Read the model definition and answer for the solid it produces. Units are mm, in the model's axes. A direction names the side the tool comes from. Give positions to 0.01 mm unless a question says otherwise; leave off trailing zeros. Loops run counter-clockwise (first coordinate to the right, second up) from the corner with the lowest first, then second, coordinate; pieces in that order, holes last. Notation, with made-up numbers: (-4, -31.5) - (48, -31.5) arc R8 cw to (48, -17.5) - close; hole circle Ø8 at (57, 73). An arc over 180 degrees is marked (long way). Put each result on its own line as item: value. Start each with the question number.
1. For faces 1 (the flat face through (3, 1.6, -2.1)), 2 (the flat face through (1, 4, -3)), 3 (the flat face through (53, 3, -17.46)), determine the directions among +Z, -Z, +X, -X, +Y, -Y from which every point of the face is accessible in a straight line to the end or side of a thin tool.
2. Consider L1, parallel to Y at x = 52.8, z = -15.81; L2, parallel to X at y = 5.5, z = -15; L3, parallel to X at y = 0.75, z = -13. Determine where each line is inside the solid, lowest interval first. Write a range as from..to.
3. A cutting plane is placed at C-C, the plane y = 0.5. Determine the outline of the cut face in (x, z).
4. A cutting plane is placed at B-B, the plane y = 3. Determine the outline of the cut face in (x, z).
5. Given pin 1 Ø3.5 at (y, z) = (3, -1.5) entering from +X; pin 2 Ø6 at (x, z) = (33, -4) entering from +Y; pin 3 Ø2 at (y, z) = (4.5, -8) entering from -X; pin 4 Ø1.2 at (y, z) = (3.5, -16) entering from -X, each flat-ended and moving along its own axis, determine where each tip first touches the part or whether it passes through.
6. A cutting plane is placed at D-D, the plane x = 34. Determine the outline of the cut face in (y, z).
7. For a pull along Y with two mould halves and no side action, classify faces 4 (the flat face through (51, 2, -15)), 5 (the flat face through (25, 0, -8)), 6 (the cylindrical face through (1.48, 2.98, -0.65)) as released by +Y, released by -Y, zero draft, split by the parting line, or undercut.
8. A cutting plane is placed at A-A, the plane z = -15.81. Determine the outline of the cut face in (x, y).
```python
from build123d import *

# Parameters (mm, degrees)
BOSS_EXTRUDE1_DEPTH = 6
SKETCH3_R           = 1
CUT_EXTRUDE1_DEPTH  = 59


with BuildPart() as part:
    # Sketch1 → Boss-Extrude1 (new body)
    with BuildSketch(Plane(origin=(0, 0, 0), x_dir=(1, 0, 0), z_dir=(0, 1, 0))):
        with BuildLine():
            Line((0, 6.17), (0, 0))
            Line((0, 0), (3, 0))
            Line((3, 0), (3, 4.33))
            ThreePointArc((3, 4.33), (3.292893219, 5.037106781), (4, 5.33))
            Line((4, 5.33), (52, 9.54))
            ThreePointArc((52, 9.54), (53.414213562, 10.125786438), (54, 11.54))
            Line((54, 11.54), (54, 17.46))
            Line((54, 17.46), (51, 17.46))
            Line((51, 17.46), (51, 13.38))
            ThreePointArc((51, 13.38), (50.707106781, 12.672893219), (50, 12.38))
            Line((50, 12.38), (2, 8.17))
            ThreePointArc((2, 8.17), (0.585786438, 7.584213562), (0, 6.17))
        make_face()
    extrude(amount=BOSS_EXTRUDE1_DEPTH)

    # Sketch3 → Cut-Extrude1 (cut)
    with BuildSketch(Plane(origin=(0, 0, 0), x_dir=(0, 0, -1), z_dir=(1, 0, 0))):
        with Locations(Location((15.81, 3, 0), (0, 0, 180))):
            Circle(SKETCH3_R)
        with BuildLine():
            Line((1.65, 4), (3.65, 4))
            ThreePointArc((3.65, 4), (4.65, 3), (3.65, 2))
            Line((3.65, 2), (1.65, 2))
            ThreePointArc((1.65, 2), (0.65, 3), (1.65, 4))
        make_face()
    extrude(amount=CUT_EXTRUDE1_DEPTH, mode=Mode.SUBTRACT)


solid = part.part
```
Return value:
1. face 1: +Z, +X, +Y, -Y
1. face 2: +X, -X
1. face 3: -Z, +X, -X, +Y, -Y
2. L1: y = 0..2, 4..6
2. L2: x = 51..54
2. L3: x = 50.92..54
3. outline: (0, -6.17) arc R2 ccw to (2, -8.17) - (50, -12.38) arc R1 cw to (51, -13.38) - (51, -17.46) - (54, -17.46) - (54, -11.54) arc R2 ccw to (52, -9.54) - (4, -5.33) arc R1 cw to (3, -4.33) - (3, 0) - (0, 0) - close
4. outline: (0, -6.17) arc R2 ccw to (2, -8.17) - (50, -12.38) arc R1 cw to (51, -13.38) - (51, -14.81) - (54, -14.81) - (54, -11.54) arc R2 ccw to (52, -9.54) - (4, -5.33) arc R1 cw to (3.05, -4.65) - (0, -4.65) - close; (0, -0.65) - (3, -0.65) - (3, 0) - (0, 0) - close; (51, -17.46) - (54, -17.46) - (54, -16.81) - (51, -16.81) - close
5. pin 1: stops at x = 3
5. pin 2: passes through
5. pin 3: stops at x = 0.18
5. pin 4: stops at x = 51
6. outline: (0, -10.98) - (6, -10.98) - (6, -7.96) - (0, -7.96) - close
7. face 4: zero draft
7. face 5: released by -Y
7. face 6: undercut
8. outline: (51, 0) - (54, 0) - (54, 2) - (51, 2) - close; (51, 4) - (54, 4) - (54, 6) - (51, 6) - close
